Read the model definition and answer for the solid it produces. Units are mm, in the model's axes. A direction names the side the tool comes from. Round coordinates to 2 decimals unless told otherwise and drop trailing zeros. Write each loop counter-clockwise with the first axis right and the second up, starting at its lowest first coordinate (ties: lowest second). Pieces come first, ordered by that corner, then holes. Notation, with made-up numbers: (27.5, -21.75) -> (62.5, -21.75) arc R26 ccw to (62.5, -0.75) -> close; hole circle Ø7 at (6.25, 30.25). An arc over 180 degrees is marked (long way). Return JSON: item names as keys, results as strings.
from build123d import *

# Parameters (mm, degrees)
SKETCH_1_W             = 38
SKETCH_1_H             = 21
EXTRUDE_1_DEPTH        = 3
SKETCH_2_R             = 1.3
CUT_EXTRUDE_1_DEPTH    = 3
PATTERN_LINEAR_1_COUNT = 2
PATTERN_LINEAR_1_PITCH = 24
SKETCH_3_W             = 15
SKETCH_3_H             = 21
EXTRUDE_2_DEPTH        = 15
SKETCH_4_W             = 5
SKETCH_4_H             = 21
EXTRUDE_3_DEPTH        = 60
SKETCH_5_R             = 2.5
CUT_EXTRUDE_2_DEPTH    = 60
FILLET_1_R             = 10.5


with BuildPart() as part:
    # 草图1 → 凸台-拉伸1 (new body)
    with BuildSketch(Plane.XY):
        with Locations((-8.78974359, -2.405128205)):
            Rectangle(SKETCH_1_W, SKETCH_1_H)
    extrude(amount=EXTRUDE_1_DEPTH)

    # 草图2 → 切除-拉伸1 (cut)
    with BuildSketch(Plane.XY.offset(3)):
        with Locations((-20.78974359, 3.594871795)):
            Circle(SKETCH_2_R)
        with Locations((-20.78974359, -8.405128205)):
            Circle(SKETCH_2_R)
    cut_extrude_1 = extrude(amount=-CUT_EXTRUDE_1_DEPTH, mode=Mode.SUBTRACT)

    # 阵列(线性)1: 切除-拉伸1 ×2
    with Locations(*[(i * PATTERN_LINEAR_1_PITCH, 0, 0) for i in range(1, PATTERN_LINEAR_1_COUNT)]):
        add(cut_extrude_1, mode=Mode.SUBTRACT)

    # 草图3 → 凸台-拉伸2 (add)
    with BuildSketch(Plane.XY.offset(3)):
        with Locations((-8.78974359, -2.405128205)):
            Rectangle(SKETCH_3_W, SKETCH_3_H)
    extrude(amount=EXTRUDE_2_DEPTH)

    # 草图4 → 凸台-拉伸3 (add)
    with BuildSketch(Plane.XY.offset(18)):
        with Locations((-8.78974359, -2.405128205)):
            Rectangle(SKETCH_4_W, SKETCH_4_H)
    extrude(amount=EXTRUDE_3_DEPTH)

    # 草图5 → 切除-拉伸2 (cut)
    with BuildSketch(Plane(origin=(-6.28974359, 0, 0), x_dir=(0, 0, -1), z_dir=(1, 0, 0))):
        with Locations(Location((-68, -2.405128205, 0), (0, 0, 90))):
            Circle(SKETCH_5_R)
    extrude(amount=-CUT_EXTRUDE_2_DEPTH, mode=Mode.SUBTRACT)

    # 圆角1
    fillet_1_edges = [part.edges().sort_by_distance(p)[0] for p in [
        (-8.78974359, 8.094871795, 78),
        (-8.78974359, -12.905128205, 78),
    ]]
    fillet(fillet_1_edges, radius=FILLET_1_R - 0.0001)  # a hair under: the kernel refuses the full size


solid = part.part
Item 1: Section B-B (y = -6) is taken. Give the vertices of the cut face in (x, z), then the cut area to 3 significant figures.
Worked answers:
{"outline": "(-27.79, 0) -> (10.21, 0) -> (10.21, 3) -> (-1.29, 3) -> (-1.29, 18) -> (-6.29, 18) -> (-6.29, 77.37) -> (-11.29, 77.37) -> (-11.29, 18) -> (-16.29, 18) -> (-16.29, 3) -> (-27.79, 3) -> close", "area": "636 mm2"}
Item 2: For a pull along Y with two mould halves and no side action, classify faces 1 (the cylindrical face through (-19.55, -8.01, 1.52)), 2 (the flat face through (-1.29, -3, 10)), 3 (the cylindrical face through (2.25, 4.47, 1.52)), 4 (the flat face through (-9, -12.905, 21)) as released by +Y, released by -Y, zero draft, split by the parting line, or undercut.
Worked answers:
{"face 1": "undercut", "face 2": "zero draft", "face 3": "undercut", "face 4": "released by -Y"}
Item 3: Flat-ended cylindrical pins translate along their axes: pin 1 (8 mm diameter, centred on x = -8, y = -7, fed in from +Z); pin 2 (9 mm diameter, centred on x = -23, y = 0.5, fed in from +Z); pin 3 (4.5 mm diameter, centred on y = 0.5, z = 14, fed in from -X). Find the tip coordinate at first contact, or state that the pin passes through.
Worked answers:
{"pin 1": "stops at z = 77.98", "pin 2": "stops at z = 3", "pin 3": "stops at x = -16.29"}
Item 4: Section C-C (z = 24) is taken. Give the vertices of the cut face in (x, y), then the cut area to 3 significant figures.
Worked answers:
{"outline": "(-11.29, -12.91) -> (-6.29, -12.91) -> (-6.29, 8.09) -> (-11.29, 8.09) -> close", "area": "105 mm2"}
Item 5: Section D-D (x = -3.5) is taken. Give the vertices of the cut face in (y, z).
Worked answers:
{"outline": "(-12.91, 0) -> (8.09, 0) -> (8.09, 18) -> (-12.91, 18) -> close"}
Item 6: Straight lines are drawn through the part: L1, parallel to Z at x = 5, y = -4.5; L2, parallel to Z at x = -5.5, y = 6; L3, parallel to X at y = -8, z = 61.5. For each, find the intervals that lie inside material, in ascending order. Write a range as [from, to].
Worked answers:
{"L1": "z = [0, 3]", "L2": "z = [0, 18]", "L3": "x = [-11.29, -6.29]"}
Item 7: A tool of negligible diameter and unlimited length cuts with its end or side. For faces 5 (the flat face through (-14, -2, 18)), 6 (the flat face through (4, -2, 3)), 7 (the cylindrical face through (-8.755, -9.911, 74.843)), from which of +Z, -Z, +X, -X, +Y, -Y can it reach the whole face along a straight path? Write none if from no direction.
Worked answers:
{"face 5": "+Z, -X, +Y, -Y", "face 6": "+Z, +X, +Y, -Y", "face 7": "+Z, +X, -X, -Y"}
